from build123d import *

# Parameters (mm, degrees)
SKETCH_1_R      = 16
SKETCH_1_R_2    = 11
EXTRUDE_1_DEPTH = 4
SKETCH_2_R      = 28
SKETCH_2_R_2    = 13
EXTRUDE_2_DEPTH = 3
EXTRUDE_3_DEPTH = 20


with BuildPart() as part:
    # 草图1 → 凸台-拉伸1 (new body)
    with BuildSketch(Plane.XY):
        Circle(SKETCH_1_R)
        Circle(SKETCH_1_R_2, mode=Mode.SUBTRACT)
    extrude(amount=EXTRUDE_1_DEPTH)

    # 草图2 → 凸台-拉伸2 (add)
    with BuildSketch(Plane.XY.offset(4)):
        Circle(SKETCH_2_R)
        Circle(SKETCH_2_R_2, mode=Mode.SUBTRACT)
    extrude(amount=EXTRUDE_2_DEPTH)

    # 草图3 → 凸台-拉伸3 (add)
    with BuildSketch(Plane.XY.offset(7)):
        with BuildLine():
            Line((-8.892523726, 24.43200814), (-6.498382723, 17.854159795))
            ThreePointArc((-6.498382723, 17.854159795), (0, 19), (6.498382723, 17.854159795))
            Line((6.498382723, 17.854159795), (8.892523726, 24.43200814))
            ThreePointArc((8.892523726, 24.43200814), (0, 26), (-8.892523726, 24.43200814))
        make_face()
        with BuildLine():
            Line((24.43200814, 8.892523726), (17.854159795, 6.498382723))
            ThreePointArc((17.854159795, 6.498382723), (19, 0), (17.854159795, -6.498382723))
            Line((17.854159795, -6.498382723), (24.43200814, -8.892523726))
            ThreePointArc((24.43200814, -8.892523726), (26, 0), (24.43200814, 8.892523726))
        make_face()
        with BuildLine():
            Line((8.892523726, -24.43200814), (6.498382723, -17.854159795))
            ThreePointArc((6.498382723, -17.854159795), (0, -19), (-6.498382723, -17.854159795))
            Line((-6.498382723, -17.854159795), (-8.892523726, -24.43200814))
            ThreePointArc((-8.892523726, -24.43200814), (0, -26), (8.892523726, -24.43200814))
        make_face()
        with BuildLine():
            Line((-24.43200814, -8.892523726), (-17.854159795, -6.498382723))
            ThreePointArc((-17.854159795, -6.498382723), (-19, 0), (-17.854159795, 6.498382723))
            Line((-17.854159795, 6.498382723), (-24.43200814, 8.892523726))
            ThreePointArc((-24.43200814, 8.892523726), (-26, 0), (-24.43200814, -8.892523726))
        make_face()
    extrude(amount=EXTRUDE_3_DEPTH)


solid = part.part
The listing builds one solid part. Answer for the finished solid, in the listing's coordinates (mm). A direction names the side the tool comes from. Round coordinates to 2 decimals unless told otherwise and drop trailing zeros. Order: outer loops, then holes, each group sorted by start corner. A loop starts at its lowest first (then second) coordinate and runs counter-clockwise, first axis right, second up. Notation, with made-up numbers: M -24.75,78 L -15.75,78 A22 cw -15.75,111 Z; hole C 45.25,41 d1. An arc over 180 degrees is marked long. Answer in a Markdown table with one row per item. Add a question column.
1) Which of the six approach directions +Z, -Z, +X, -X, +Y, -Y give full straight-line access (tool end or side, diameter ignored) to faces 1 (the face through (7.712, -21.189, 16.86)), 2 (the face through (-22, 0, 27)), 3 (the face through (-26, 0, 17)), 4 (the face through (-21.189, -7.712, 16.86)), 5 (the face through (19, 0, 17))?
2) The part is cut by section B-B on z = 20.5. Determine the outline of the cut face in (x, y), plus the area to 3 significant figures.
3) The part is cut by section A-A on x = 0. Determine the outline of the cut face in (y, z).
4) Flat-ended cylindrical pins translate along their axes: pin 1 Ø3 at (y, z) = (22, 3.5) entering from +X; pin 2 Ø1 at (x, z) = (17, 10.5) entering from +Y; pin 3 Ø2 at (x, z) = (-20, 10) entering from +Y; pin 4 Ø1.5 at (y, z) = (-0.5, 15) entering from -X. Find the tip coordinate at first contact, or state that the pin passes through.
5) Consider line 1 along Y through (x, z) = (0, 2.55); line 2 along Y through (x, z) = (0, 5.95); line 3 along Z through (x, y) = (14.5, -19). Determine where each line is inside the solid, lowest interval first. Write a range as from..to.
6) Determine the mould class of faces 6 (the face through (-11, 3, 4)), 7 (the face through (12, -12, 4)), 8 (the face through (0, 26, 17)), 9 (the face through (21.1, -7.68, 16.86)) for opening direction Y: pulls with the +Y half, pulls with the -Y half, needs draft (parallel to the pull), parting line crosses it, or undercut.
7) The part is cut by section D-D on y = -14.5. Determine the outline of the cut face in (x, z), plus the area to 3 significant figures.
Findings below:
| question | item | result |
|---|---|---|
| 1 | face 1 | +Z, +X |
| 1 | face 2 | +Z, +X, -X, +Y, -Y |
| 1 | face 3 | +Z, -X |
| 1 | face 4 | +Z, -Y |
| 1 | face 5 | +Z |
| 2 | outline | M -24.43,-8.89 L -17.85,-6.5 A19 cw -17.85,6.5 L -24.43,8.89 A26 ccw Z; M -8.89,-24.43 A26 ccw 8.89,-24.43 L 6.5,-17.85 A19 cw -6.5,-17.85 Z; M -8.89,24.43 L -6.5,17.85 A19 cw 6.5,17.85 L 8.89,24.43 A26 ccw Z; M 17.85,-6.5 L 24.43,-8.89 A26 ccw 24.43,8.89 L 17.85,6.5 A19 cw Z |
| 2 | area | 440 mm² |
| 3 | outline | M -28,4 L -16,4 L -16,0 L -11,0 L -11,4 L -13,4 L -13,7 L -19,7 L -19,27 L -26,27 L -26,7 L -28,7 Z; M 11,0 L 16,0 L 16,4 L 28,4 L 28,7 L 26,7 L 26,27 L 19,27 L 19,7 L 13,7 L 13,4 L 11,4 Z |
| 4 | pin 1 | stops at x = 18.98 |
| 4 | pin 2 | passes through |
| 4 | pin 3 | stops at y = 7.64 |
| 4 | pin 4 | stops at x = -26 |
| 5 | line 1 | y = -16..-11, 11..16 |
| 5 | line 2 | y = -28..-13, 13..28 |
| 5 | line 3 | z = 4..7 |
| 6 | face 6 | undercut |
| 6 | face 7 | needs draft |
| 6 | face 8 | pulls with the +Y half |
| 6 | face 9 | pulls with the -Y half |
| 7 | outline | M -23.95,4 L -6.76,4 L -6.76,0 L 6.76,0 L 6.76,4 L 23.95,4 L 23.95,7 L -23.95,7 Z |
| 7 | area | 198 mm² |
